from build123d import *

# Parameters (mm, degrees)
SKETCH1_R           = 25.4
SKETCH1_R_2         = 21.4
BOSS_EXTRUDE1_DEPTH = 28
SKETCH2_R           = 21.4
BOSS_EXTRUDE3_DEPTH = 5
FILLET3_R           = 2
FILLET4_R           = 1
FILLET5_R           = 0.5


with BuildPart() as part:
    # Sketch1 → Boss-Extrude1 (new body)
    with BuildSketch(Plane.XY):
        Circle(SKETCH1_R)
        Circle(SKETCH1_R_2, mode=Mode.SUBTRACT)
    extrude(amount=BOSS_EXTRUDE1_DEPTH)

    # Sketch2 → Boss-Extrude3 (add)
    with BuildSketch(Plane.XY.offset(28)):
        Circle(SKETCH2_R)
    extrude(amount=-BOSS_EXTRUDE3_DEPTH)

    # Fillet3
    fillet3_edges = [part.edges().sort_by_distance(p)[0] for p in [
        (-21.4, 0, 0),
    ]]
    fillet(fillet3_edges, radius=FILLET3_R)

    # Fillet4
    fillet4_edges = [part.edges().sort_by_distance(p)[0] for p in [
        (-25.4, 0, 0),
    ]]
    fillet(fillet4_edges, radius=FILLET4_R)

    # Fillet5
    fillet5_edges = [part.edges().sort_by_distance(p)[0] for p in [
        (-25.4, 0, 28),
    ]]
    fillet(fillet5_edges, radius=FILLET5_R)


solid = part.part
Here's how the part is built. I have some questions about the finished solid (model axes, mm). A direction names the side the tool comes from. Coordinates: 2 decimals unless noted, no trailing zeros. Order: outer loops, then holes, each group sorted by start corner. A loop starts at its lowest first (then second) coordinate and runs counter-clockwise, first axis right, second up.
Item 1: If we section it at D-D on z = 24: List the corners of the cut face in (x, y) for me.
Result sheet:
outline: circle Ø50.8 at (0, 0)
Item 2: For faces 1 (the face through (13, -20, 0)), 2 (the face through (-4.6, -20.9, 12.4)), which set-ups out of +Z, -Z, +X, -X, +Y, -Y let a thin tool reach every point of the face, with its end or its side?
Result sheet:
face 1: -Z, +X, -X, +Y, -Y
face 2: -Z
Item 3: If we section it at C-C on z = 20.25: List the corners of the cut face in (x, y) for me.
Result sheet:
outline: circle Ø50.8 at (0, 0); hole circle Ø42.8 at (0, 0)
Item 4: For P1, Ø10, axis at x = 7, z = 16, coming from the +Y side; P2, Ø13, axis at x = 10.5, y = 6, coming from the -Z side; P3, Ø10, axis at x = 9.5, z = 14, coming from the +Y side, each with a flat end and sliding along its axis, tell me the tip position at first contact or that it passes through.
Result sheet:
P1: stops at y = 25.32
P2: stops at z = 23
P3: stops at y = 25
Item 5: I need wall thicknesses on line 1 (Y direction, x = 0, z = 11); line 2 (Z direction, x = 15.5, y = -2); line 3 (X direction, y = -3, z = 10.5). Which ranges of each line are inside material? Lowest first, please.
Result sheet:
line 1: y = -25.4 to -21.4, 21.4 to 25.4
line 2: z = 23 to 28
line 3: x = -25.22 to -21.19, 21.19 to 25.22
Item 6: If we section it at A-A on y = 0: List the corners of the cut face in (x, z) for me, plus the area to 3 significant figures.
Result sheet:
outline: (-25.4, 1) arc R1 ccw to (-24.4, 0) - (-23.4, 0) arc R2 ccw to (-21.4, 2) - (-21.4, 23) - (21.4, 23) - (21.4, 2) arc R2 ccw to (23.4, 0) - (24.4, 0) arc R1 ccw to (25.4, 1) - (25.4, 27.5) arc R0.5 ccw to (24.9, 28) - (-24.9, 28) arc R0.5 ccw to (-25.4, 27.5) - close
area: 436 mm2
Item 7: If we mould it in two halves opening along Y, with no side actions, what happens to faces 3 (the face through (-5.506, -24.796, 14.064)), 4 (the face through (0, 0, 28)), 5 (the face through (0, 0, 23))? For each: +Y half, -Y half, draft (parallel to the pull), parting line (faces both ways), or undercut.
Result sheet:
face 3: parting line
face 4: draft
face 5: undercut
